Work out the finished part from the listing and answer in its coordinate system (mm). Coordinates: 2 decimals unless noted, no trailing zeros. Write item = value, one per line. Start each with the question number.
Q1. For a pull along Y with two mould halves and no side action, classify faces 1 (the flat face through (1, 1, 0)), 2 (the cylindrical face through (34.481, -102.397, -0.76)) as +Y half, -Y half, draft (parallel to the pull), parting line (faces both ways), or undercut.
Q2. Straight lines are drawn through the part: L1, parallel to X at y = -48, z = -0.5; L2, parallel to X at y = 100.75, z = -1.1; L3, parallel to Y at x = 30, z = -0.6. For each, find the intervals that lie inside material, in ascending order. Write a range as from..to.
Q3. Flat-ended cylindrical pins translate along their axes: pin 1 (4.5 mm diameter, centred on x = 35, y = 100.75, fed in from +Z); pin 2 (3 mm diameter, centred on x = -35, y = -100.75, fed in from -Z). Find the tip coordinate at first contact, or state that the pin passes through.
Autodesk Inventor part; units mm, degrees
ref_plane "YZ Plane" through (0, 0, 0) normal (1, 0, 0) x (0, 1, 0)
ref_plane "XZ Plane" through (0, 0, 0) normal (0, 1, 0) x (-1, 0, 0)
ref_plane "XY Plane" through (0, 0, 0) normal (0, 0, 1) x (1, 0, 0)
sketch "Sketch1" plane through (0, 0, 0) normal (0, 0, 1) x (1, 0, 0)
  line L0 (-41.5, 48) -> (41.5, 48)
  line L1 (41.5, 48) -> (41.5, -48)
  line L2 (41.5, -48) -> (-41.5, -48)
  line L3 (-41.5, -48) -> (-41.5, 48)
  point P0 (0, 0)
  dimension "d0" = 83
  dimension "d1" = 96
  dimension "d2" = 48
  dimension "d3" = 41.5
extrude "Extrusion1" add sketch "Sketch1" against normal blind 1.5
sketch "Sketch7" plane through (-41.5, 48, 0) normal (0, 1, 0) x (1, 0, 0)
  line L0 (0, 0) -> (83, 0)
  line L1 (83, 0) -> (83, 1.5)
  line L2 (0, 1.5) -> (83, 1.5)
  line L3 (0, 0) -> (0, 1.5)
  point P0 (41.5, 0)
extrude "Extrusion5" add sketch "Sketch7" along normal blind 56.75
sketch "Sketch8" plane through (-41.5, -48, 0) normal (0, -1, 0) x (1, 0, 0)
  line L0 (83, 0) -> (0, 0)
  line L1 (0, 0) -> (0, -1.5)
  line L2 (83, -1.5) -> (0, -1.5)
  line L3 (83, 0) -> (83, -1.5)
  point P0 (41.5, 0)
extrude "Extrusion6" add sketch "Sketch8" along normal blind 56.75
sketch "Sketch9" plane through (0, 0, 0) normal (0, 0, 1) x (1, 0, 0)
  circle A0 centre (35, -100.75) radius 3
  circle A1 centre (-35, -100.75) radius 3
  circle A2 centre (-30, -48) radius 3
  circle A3 centre (30, -48) radius 3
  circle A4 centre (30, 48) radius 3
  circle A5 centre (-30, 48) radius 3
  circle A6 centre (35, 100.75) radius 3
  circle A7 centre (-35, 100.75) radius 3
  point P0 (0, 0)
hole "Hole3" at (35, -100.75, 0) at (-35, -100.75, 0) at (30, -48, 0) at (-30, -48, 0) at (30, 48, 0) at (-30, 48, 0) at (35, 100.75, 0) at (-35, 100.75, 0) direction (0, 0, -1) diameter 3.454 end through all
properties part number "memesat shear panel type 2" material "Aluminum 6061"
Model answer:
q1.face_1 = draft
q1.face_2 = undercut
q2.L1 = -41.5..-31.73, -28.27..28.27, 31.73..41.5
q2.L2 = -41.5..-36.73, -33.27..33.27, 36.73..41.5
q2.L3 = -104.75..-49.73, -46.27..46.27, 49.73..104.75
q3.pin_1 = 0
q3.pin_2 = through
